For this review, take the finished solid that the model builds, in its own axes (mm). A direction names the side the tool comes from. Coordinates: 2 decimals unless noted, no trailing zeros. Write each loop counter-clockwise with the first axis right and the second up, starting at its lowest first coordinate (ties: lowest second). Pieces come first, ordered by that corner, then holes.
1) Mouldability with a two-part tool opening along Z and no side actions: class faces 3 (the face through (-1, -30.48, 24)), 4 (the face through (95.334, -19.593, -30.022)), 5 (the face through (21.804, 28.114, -6.867)) as pulls with the +Z half, pulls with the -Z half, needs draft (parallel to the pull), parting line crosses it, or undercut.
2) Insertion check: P1, Ø1, axis at y = 53.5, z = 28.5, coming from the +X side; P2, Ø10, axis at x = -16.5, y = 23, coming from the -Z side; P3, Ø8, axis at x = 21.5, y = 38.5, coming from the +Z side. Each pin has a flat end and moves straight along its axis. Give the tip position at first contact, or say it passes through.
3) We need section B-B on y = 36.5. Write out the cut boundary in (x, z).
4) To check wall thickness, follow line 1 along Z through (x, y) = (0, 21.5); line 2 along X through (y, z) = (43, 0); line 3 along X through (y, z) = (-2, 0). State the ranges of each line that lie inside material, in increasing order.
5) For faces 1 (the face through (-1, 85.09, -24)), 2 (the face through (69.64, 27.1, 53.4)), list the 3-axis set-ups (+Z, -Z, +X, -X, +Y, -Y) from which the entire face can be reached by the end or side of a thin tool; tool diameter is ignored.
6) We need section A-A on y = 70. Write out the cut boundary in (x, z).
Autodesk Inventor part; units mm, degrees
ref_plane "YZ Plane" through (0, 0, 0) normal (1, 0, 0) x (0, 1, 0)
ref_plane "XZ Plane" through (0, 0, 0) normal (0, 1, 0) x (-1, 0, 0)
ref_plane "XY Plane" through (0, 0, 0) normal (0, 0, 1) x (1, 0, 0)
sketch "Sketch1" plane through (0, 0, 0) normal (0, 1, 0) x (-1, 0, 0)
  circle A0 centre (0, 0) radius 87.757
  dimension "d0" = 175.514
extrude "Extrusion1" add sketch "Sketch1" along normal blind 54.61
sketch "Sketch2" plane through (0, 54.61, 0) normal (0, 1, 0) x (1, 0, 0)
  circle A0 centre (0, 0) radius 99.949
  dimension "d3" = 199.898
sketch "Sketch3" plane through (0, 0, 0) normal (0, -1, 0) x (1, 0, 0)
  circle A0 centre (0, 0) radius 99.949
  dimension "d4" = 199.898
extrude "Extrusion2" add sketch "Sketch2" along normal blind 30.48
extrude "Extrusion3" add sketch "Sketch3" along normal blind 30.48
sketch "Sketch4" plane through (0, 85.09, 0) normal (0, 1, 0) x (1, 0, 0)
  circle A0 centre (0, 0) radius 22.86
  dimension "d9" = 45.72
extrude "Extrusion4" cut sketch "Sketch4" against normal blind 115.57
fillet "Fillet1" radius 12.7 1 edges at (87.757, 54.61, 0)
fillet "Fillet2" radius 12.7 1 edges at (87.757, 0, 0)
fillet "Fillet3" radius 12.7 4 edges at (0, 0, 99.949) (0, 0, -99.949) (0, 54.5998, 99.949) (0, 54.5998, -99.949)
properties part number "Pulley" material "Acetal Resin, Black"
Result:
1. face 3: needs draft
1. face 4: parting line crosses it
1. face 5: undercut
2. P1: stops at x = 91.23
2. P2: stops at z = -87
2. P3: stops at z = 85.99
3. outline: circle Ø175.51 at (0, 0); hole circle Ø45.72 at (0, 0)
4. line 1: z = -87.76 to -22.86, 22.86 to 87.76
4. line 2: x = -87.8 to -22.86, 22.86 to 87.8
4. line 3: x = -97.84 to -22.86, 22.86 to 97.84
5. face 1: +Z, -Z, +X, -X, +Y
5. face 2: none
6. outline: circle Ø199.9 at (0, 0); hole circle Ø45.72 at (0, 0)
